```python
from build123d import *

# Parameters (mm, degrees)
SKETCH1_R           = 10
BOSS_EXTRUDE1_DEPTH = 138.8
SKETCH2_R           = 7
BOSS_EXTRUDE2_DEPTH = 71
CUT_EXTRUDE1_DEPTH  = 3
CUT_EXTRUDE2_DEPTH  = 3.5


with BuildPart() as part:
    # Sketch1 → Boss-Extrude1 (new, symmetric)
    with BuildSketch(Plane.XY):
        Circle(SKETCH1_R)
    extrude(amount=BOSS_EXTRUDE1_DEPTH, both=True)

    # Sketch2 → Boss-Extrude2 (add)
    with BuildSketch(Plane.XY.offset(138.8)):
        Circle(SKETCH2_R)
    extrude(amount=BOSS_EXTRUDE2_DEPTH)

    # Sketch4 → Cut-Extrude1 (cut)
    with BuildSketch(Plane(origin=(0, 7, 0), x_dir=(1, 0, 0), z_dir=(0, 1, 0))):
        with BuildLine():
            Line((-2.5, -197.8), (-2.5, -157.8))
            ThreePointArc((-2.5, -157.8), (0, -155.3), (2.5, -157.8))
            Line((2.5, -157.8), (2.5, -197.8))
            ThreePointArc((2.5, -197.8), (0, -200.3), (-2.5, -197.8))
        make_face()
    extrude(amount=-CUT_EXTRUDE1_DEPTH, mode=Mode.SUBTRACT)

    # Sketch5 → Cut-Extrude2 (cut)
    with BuildSketch(Plane(origin=(0, 10, 0), x_dir=(1, 0, 0), z_dir=(0, 1, 0))):
        with BuildLine():
            Line((-3, -40), (-3, 40))
            ThreePointArc((-3, 40), (0, 43), (3, 40))
            Line((3, 40), (3, -40))
            ThreePointArc((3, -40), (0, -43), (-3, -40))
        make_face()
    extrude(amount=-CUT_EXTRUDE2_DEPTH, mode=Mode.SUBTRACT)


solid = part.part
```
Check sheet for the modelled part. Datum: model origin and axes. Units: mm. A direction names the side the tool comes from. Give positions to 0.01 mm unless a question says otherwise; leave off trailing zeros. Order: outer loops, then holes, each group sorted by start corner. A loop starts at its lowest first (then second) coordinate and runs counter-clockwise, first axis right, second up. Notation, with made-up numbers: (-8.75, 19.25) -> (31.25, 19.25) arc R16 cw to (31.25, 27.25) -> close; hole circle Ø3 at (40, 8.25). An arc over 180 degrees is marked (long way). Return JSON: item names as keys, results as strings.
1. Go/stop test with flat-tipped pins: P1, Ø10, axis at y = -7, z = 101.5, coming from the -X side; P2, Ø1, axis at y = 5, z = 4.5, coming from the +X side; P3, Ø3, axis at x = 1, z = 12.5, coming from the +Y side. Record where each tip stops, or that it passes through.
From the geometry:
{"P1": "x = -9.8", "P2": "x = 8.93", "P3": "y = 6.5"}
2. Mould release check, pull along Z, two halves, no side actions. Record for faces 1 (the flat face through (0, 0, 209.8)), 2 (the flat face through (0, 0, -138.8)), 3 (the cylindrical face through (-1.517, -6.834, 173.803)), 4 (the flat face through (0, 6.5, -1)): +Z half, -Z half, draft (parallel to the pull), parting line (faces both ways), or undercut.
From the geometry:
{"face 1": "+Z half", "face 2": "-Z half", "face 3": "draft", "face 4": "undercut"}
3. Material ranges on probe 1 along Z at (x, y) = (2.5, -8.5); probe 2 along Z at (x, y) = (1, 7.5); probe 3 along Y at (x, z) = (-1, -19), recorded low to high. Write a range as [from, to].
From the geometry:
{"probe 1": "[-138.8, 138.8]", "probe 2": "[-138.8, -42.83], [42.83, 138.8]", "probe 3": "[-9.95, 6.5]"}
4. Cross-section at A-A, the plane y = 0. Record the cut outline in (x, z).
From the geometry:
{"outline": "(-10, -138.8) -> (10, -138.8) -> (10, 138.8) -> (7, 138.8) -> (7, 209.8) -> (-7, 209.8) -> (-7, 138.8) -> (-10, 138.8) -> close"}
5. Set-up check for faces 5 (the cylindrical face through (-2.17, -9.76, 1.94)), 6 (the flat face through (-7, -2, 138.8)): record each of +Z, -Z, +X, -X, +Y, -Y from which the full face is reachable in a straight line by a thin tool's end or side.
From the geometry:
{"face 5": "+Z, -Z", "face 6": "+Z"}
6. Cross-section at B-B, the plane z = 24. Record the cut outline in (x, y).
From the geometry:
{"outline": "(-3, 6.5) -> (-3, 9.54) arc R10 ccw (long way) to (3, 9.54) -> (3, 6.5) -> close"}
